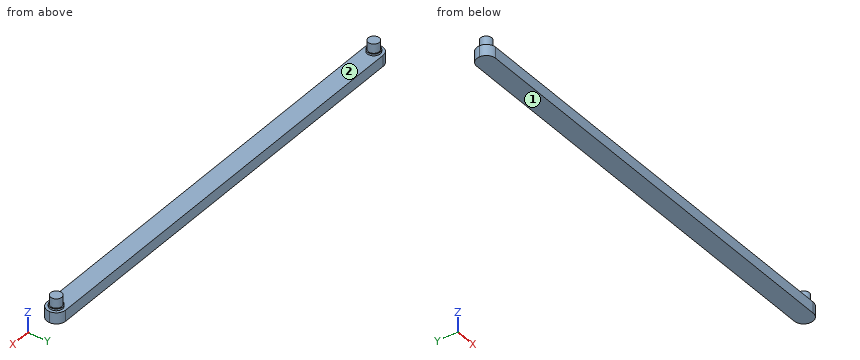
from build123d import *

# Parameters (mm, degrees)
SKETCH1_W            = 122.5
SKETCH1_H            = 10.198852772
BOSS_EXTRUDE1_DEPTH  = 6
FILLET1_R            = 5
SKETCH2_R            = 3.5
BOSS_EXTRUDE2_DEPTH  = 1
SKETCH3_R            = 3
BOSS_EXTRUDE3_DEPTH  = 5
FILLET1_OF_MIRROR1_R = 5


with BuildPart() as part:
    # Sketch1 → Boss-Extrude1 (new body)
    with BuildSketch(Plane.XY):
        Rectangle(SKETCH1_W, SKETCH1_H)
    boss_extrude1 = extrude(amount=BOSS_EXTRUDE1_DEPTH)

    # Fillet1
    fillet1_edges = [part.edges().sort_by_distance(p)[0] for p in [
        (61.25, -5.099426386, 3),
        (61.25, 5.099426386, 3),
    ]]
    fillet(fillet1_edges, radius=FILLET1_R)

    # Sketch2 → Boss-Extrude2 (add)
    with BuildSketch(Plane.XY.offset(6)):
        with Locations((56.25, 0)):
            Circle(SKETCH2_R)
    boss_extrude2 = extrude(amount=BOSS_EXTRUDE2_DEPTH)

    # Sketch3 → Boss-Extrude3 (add)
    with BuildSketch(Plane.XY.offset(7)):
        with Locations((56.25, 0)):
            Circle(SKETCH3_R)
    boss_extrude3 = extrude(amount=BOSS_EXTRUDE3_DEPTH)

    # Mirror1: Boss-Extrude1, Boss-Extrude2, Boss-Extrude3 across plane
    add(boss_extrude1.mirror(Plane(origin=(-61.25, 5.099426386, 6), x_dir=(0, 0, 1), z_dir=(1, 0, 0))))
    add(boss_extrude2.mirror(Plane(origin=(-61.25, 5.099426386, 6), x_dir=(0, 0, 1), z_dir=(1, 0, 0))))
    add(boss_extrude3.mirror(Plane(origin=(-61.25, 5.099426386, 6), x_dir=(0, 0, 1), z_dir=(1, 0, 0))))

    # Fillet1 of Mirror1
    fillet1_of_mirror1_edges = [part.edges().sort_by_distance(p)[0] for p in [
        (-183.75, -5.099426386, 3),
        (-183.75, 5.099426386, 3),
    ]]
    fillet(fillet1_of_mirror1_edges, radius=FILLET1_OF_MIRROR1_R)


solid = part.part
The listing builds one solid part. Answer for the finished solid, in the listing's coordinates (mm). Face numbers are marked on the shaded views. Coordinates: 2 decimals unless noted, no trailing zeros. Write each loop counter-clockwise with the first axis right and the second up, starting at its lowest first coordinate (ties: lowest second). Pieces come first, ordered by that corner, then holes. Notation, with made-up numbers: (35.25, -17.5) - (92.25, -17.5) arc R36 ccw to (92.25, 17.5) - close; hole circle Ø1 at (65, 66.5). An arc over 180 degrees is marked (long way). Put each result on its own line as item: value.
1. Determine the mould class of the marked faces 1 and 2 for opening direction X: pulls with the +X half, pulls with the -X half, needs draft (parallel to the pull), parting line crosses it, or undercut.
Answer sheet:
face 1: needs draft
face 2: undercut
2. The part is cut by section B-B on x = -132. Give the vertices of the cut face in (y, z).
Answer sheet:
outline: (-5.1, 0) - (5.1, 0) - (5.1, 6) - (-5.1, 6) - close
3. Find the intervals of material crossed by line 1 along Z through (x, y) = (-4, 1.25); line 2 along X through (y, z) = (-2.5, 6.5); line 3 along X through (y, z) = (-1.75, 1.5), in increasing order. Write a range as from..to.
Answer sheet:
line 1: z = 0..6
line 2: x = -181.2..-176.3, 53.8..58.7
line 3: x = -183.47..60.97
4. The part is cut by section A-A on z = 9. Give the vertices of the cut face in (x, y), plus the area to 3 significant figures.
Answer sheet:
outline: circle Ø6 at (-178.75, 0); circle Ø6 at (56.25, 0)
area: 56.5 mm^2
5. Flat-ended cylindrical pins translate along their axes: pin 1 Ø2 at (x, z) = (-32.5, 8) entering from -Y; pin 2 Ø1 at (y, z) = (-3.5, 7) entering from -X. Find the tip coordinate at first contact, or state that the pin passes through.
Answer sheet:
pin 1: passes through
pin 2: stops at x = -180.55
